The model under review builds one solid part; all positions refer to its coordinate system, in mm. Coordinates: 2 decimals unless noted, no trailing zeros. Loops run counter-clockwise (first coordinate to the right, second up) from the corner with the lowest first, then second, coordinate; pieces in that order, holes last. Notation, with made-up numbers: (43, -30) - (81, -30) arc R33 cw to (81, 1) - close; hole circle Ø9 at (45.25, 37.25). An arc over 180 degrees is marked (long way). Use a Markdown table: item, result. Add a question column.
1) Clearance check with flat-ended pins moving along their axes: pin 1 (10 mm diameter, centred on x = 25.5, y = -9.5, fed in from +Z); pin 2 (3 mm diameter, centred on x = 5, y = -23.5, fed in from +Z); pin 3 (6 mm diameter, centred on x = -12.5, y = -27, fed in from -Z). State where each tip first meets the part, or that it passes through.
2) To check wall thickness, follow L1, parallel to Z at x = -1.5, y = -25.5; L2, parallel to Y at x = -25.5, z = 36.5; L3, parallel to Z at x = 4, y = -34. State the ranges of each line that lie inside material, in increasing order. Write a range as [from, to].
3) Add section A-A, the plane y = -10.5. Give the boundary of the cut face in (x, z), and give its area (3 significant figures).
```python
from build123d import *

# Parameters (mm, degrees)
F0_R     = 48
F1_DEPTH = 40
F2_R     = 5
F3_R     = 5


with BuildPart() as f1:
    # F0 (on Front) → F1 (new body)
    with BuildSketch(Plane.XZ):
        Circle(F0_R)
    extrude(amount=F1_DEPTH)

    # F2
    f2_edges = [f1.edges().sort_by_distance(p)[0] for p in [
        (-48, -40, 0),
    ]]
    fillet(f2_edges, radius=F2_R)

    # F3
    f3_edges = [f1.edges().sort_by_distance(p)[0] for p in [
        (48, -17.5, 0),
        (-48, -35, 0),
        (-48, 0, 0),
    ]]
    fillet(f3_edges, radius=F3_R)


solid = f1.part
```
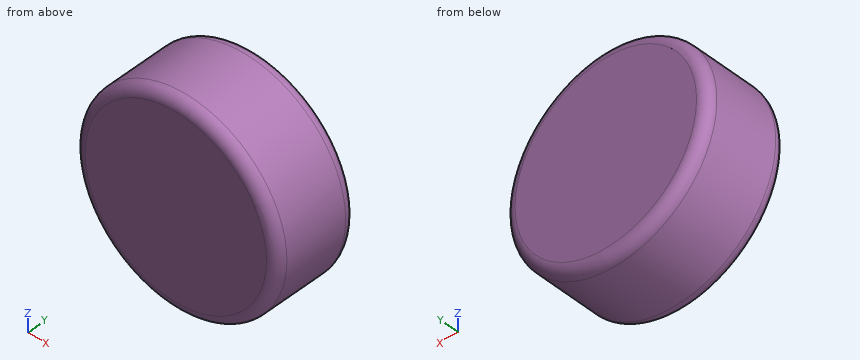
From the geometry:
| question | item | result |
|---|---|---|
| 1 | pin 1 | stops at z = 43.4 |
| 1 | pin 2 | stops at z = 47.87 |
| 1 | pin 3 | stops at z = -47.05 |
| 2 | L1 | z = [-47.98, 47.98] |
| 2 | L2 | y = [-39.76, -0.24] |
| 2 | L3 | z = [-47.83, 47.83] |
| 3 | outline | circle Ø96 at (0, 0) |
| 3 | area | 7,240 mm^2 |
